For this review, take the finished solid that the model builds, in its own axes (mm). Face numbers are marked on the shaded views. A direction names the side the tool comes from. Round coordinates to 2 decimals unless told otherwise and drop trailing zeros. Order: outer loops, then holes, each group sorted by start corner. A loop starts at its lowest first (then second) coordinate and runs counter-clockwise, first axis right, second up.
from build123d import *

# Parameters (mm, degrees)
SKETCH1_W           = 60.861702088
SKETCH1_H           = 96.997143498
BOSS_EXTRUDE1_DEPTH = 50
SKETCH2_W           = 54.597089422
SKETCH2_H           = 86.84373193
CUT_EXTRUDE1_DEPTH  = 50
SKETCH3_R           = 4.118180668
SKETCH3_R_2         = 4.272844434
SKETCH3_R_3         = 3.932739474
CUT_EXTRUDE2_DEPTH  = 6
SKETCH4_R           = 3.08771087
BOSS_EXTRUDE2_DEPTH = 2
SKETCH5_R           = 2.038212953
CUT_EXTRUDE3_DEPTH  = 2
SKETCH6_R           = 3.908744467
SKETCH6_R_2         = 2.535125685
BOSS_EXTRUDE3_DEPTH = 2
SKETCH7_R           = 2.219432532
CUT_EXTRUDE4_DEPTH  = 2
SKETCH8_W           = 47.395397398
SKETCH8_H           = 4.29160036
SKETCH8_W_2         = 46.234961005
SKETCH8_H_2         = 3.842331126
SKETCH8_W_3         = 46.458453643
SKETCH8_H_3         = 4.013838195
SKETCH8_W_4         = 44.816524007
SKETCH8_H_4         = 3.759016324
SKETCH8_W_5         = 44.332896866
SKETCH8_H_5         = 3.544111845
SKETCH8_W_6         = 43.835439371
SKETCH8_H_6         = 4.852900567
SKETCH8_W_7         = 44.232019009
SKETCH8_H_7         = 3.586032373
SKETCH8_W_8         = 44.502323157
SKETCH8_H_8         = 5.537324529
BOSS_EXTRUDE4_DEPTH = 2
SKETCH9_W           = 44.730161392
SKETCH9_H           = 4.206770637
SKETCH9_W_2         = 43.731962655
SKETCH9_H_2         = 4.51977805
BOSS_EXTRUDE5_DEPTH = 2


with BuildPart() as part:
    # Sketch1 → Boss-Extrude1 (new body)
    with BuildSketch(Plane.XY):
        Rectangle(SKETCH1_W, SKETCH1_H)
    extrude(amount=BOSS_EXTRUDE1_DEPTH)

    # Sketch2 → Cut-Extrude1 (cut)
    with BuildSketch(Plane.XY.offset(50)):
        with Locations((-0.054476232, 0.453696841)):
            Rectangle(SKETCH2_W, SKETCH2_H)
    extrude(amount=-CUT_EXTRUDE1_DEPTH, mode=Mode.SUBTRACT)

    # Sketch3 → Cut-Extrude2 (cut)
    with BuildSketch(Plane(origin=(0, 48.498571749, 0), x_dir=(1, 0, 0), z_dir=(0, 1, 0))):
        with Locations(Location((-17.379612091, -22.981855157, 0), (0, 0, 270))):
            Circle(SKETCH3_R)
        with Locations(Location((0.816264726, -22.981855157, 0), (0, 0, 270))):
            Circle(SKETCH3_R_2)
        with Locations(Location((18.098885302, -22.981855157, 0), (0, 0, 270))):
            Circle(SKETCH3_R_3)
    extrude(amount=-CUT_EXTRUDE2_DEPTH, mode=Mode.SUBTRACT)

    # Sketch4 → Boss-Extrude2 (add)
    with BuildSketch(Plane(origin=(30.430851044, 0, 0), x_dir=(0, 0, -1), z_dir=(1, 0, 0))):
        with Locations(Location((-14.163441472, 33.849346779, 0), (0, 0, 180))):
            Circle(SKETCH4_R)
    extrude(amount=BOSS_EXTRUDE2_DEPTH)

    # Sketch5 → Cut-Extrude3 (cut)
    with BuildSketch(Plane(origin=(32.430851044, 0, 0), x_dir=(0, 0, -1), z_dir=(1, 0, 0))):
        with Locations((-13.96185256, 33.734367255)):
            Circle(SKETCH5_R)
    extrude(amount=-CUT_EXTRUDE3_DEPTH, mode=Mode.SUBTRACT)

    # Sketch6 → Boss-Extrude3 (add)
    with BuildSketch(Plane.ZY.offset(30.430851044)):
        with Locations(Location((13.179644946, 35.995992558, 0), (0, 0, 180))):
            Circle(SKETCH6_R)
        with Locations((13.179644946, 35.995992558)):
            Circle(SKETCH6_R_2, mode=Mode.SUBTRACT)
    extrude(amount=BOSS_EXTRUDE3_DEPTH)

    # Sketch7 → Cut-Extrude4 (cut)
    with BuildSketch(Plane.ZY.offset(30.430851044)):
        with Locations((13.179644946, 35.995992558)):
            Circle(SKETCH7_R)
    extrude(amount=-CUT_EXTRUDE4_DEPTH, mode=Mode.SUBTRACT)

    # Sketch8 → Boss-Extrude4 (add)
    with BuildSketch(Plane.ZY.offset(-27.244068479)):
        with Locations((24.521897503, 28.206728859)):
            Rectangle(SKETCH8_W, SKETCH8_H)
        with Locations((25.229689805, 18.94599963)):
            Rectangle(SKETCH8_W_2, SKETCH8_H_2)
        with Locations((25.229689805, 10.788271288)):
            Rectangle(SKETCH8_W_3, SKETCH8_H_3)
        with Locations((23.657759327, 2.882970932)):
            Rectangle(SKETCH8_W_4, SKETCH8_H_4)
        with Locations((23.899572897, -5.013591611)):
            Rectangle(SKETCH8_W_5, SKETCH8_H_5)
        with Locations((24.148301645, -13.789703554)):
            Rectangle(SKETCH8_W_6, SKETCH8_H_6)
        with Locations((23.950011826, -21.862272303)):
            Rectangle(SKETCH8_W_7, SKETCH8_H_7)
        with Locations((24.1320976, -31.257152078)):
            Rectangle(SKETCH8_W_8, SKETCH8_H_8)
    extrude(amount=BOSS_EXTRUDE4_DEPTH)

    # Sketch9 → Boss-Extrude5 (add)
    with BuildSketch(Plane.ZY.offset(-27.244068479)):
        with Locations((24.880043499, 35.759572617)):
            Rectangle(SKETCH9_W, SKETCH9_H)
        with Locations((23.711117662, -38.822738944)):
            Rectangle(SKETCH9_W_2, SKETCH9_H_2)
    extrude(amount=BOSS_EXTRUDE5_DEPTH)


solid = part.part
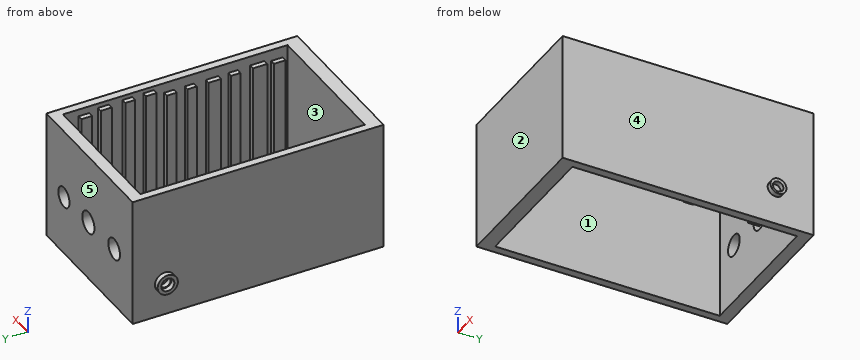
(1) Clearance check with flat-ended pins moving along their axes: P1, Ø2, axis at x = 26, y = 28, coming from the +Z side; P2, Ø4.5, axis at y = -30.5, z = 23.5, coming from the -X side; P3, Ø1, axis at x = 26.5, y = -39.5, coming from the -Z side. State where each tip first meets the part, or that it passes through.
(2) Tool access review of the marked faces 1 and 2: name each direction out of +Z, -Z, +X, -X, +Y, -Y from which nothing blocks a thin tool from reaching the whole face with its end or side.
(3) Wall thickness on L1, parallel to Y at x = 23, z = 41; L2, parallel to X at y = 10, z = 44.5; L3, parallel to X at y = -7, z = 37: over which ranges is each line inside the solid? List them lowest first.
(4) Add section B-B on x = -8. Give the boundary of the cut face in (y, z).
(5) Add section A-A on y = 24.5. Give the boundary of the cut face in (x, z).
(6) Add section D-D on x = -16. Give the boundary of the cut face in (y, z), plus the area to 3 significant figures.
(7) Add section C-C on y = -14. Give the boundary of the cut face in (x, z).
(8) Draft analysis for pull direction Y (two halves, no side actions). For the marked faces 3, 4 and 5, state which applies: pulls with the +Y half, pulls with the -Y half, needs draft (parallel to the pull), parting line crosses it, or undercut.
Here are the results:
1. P1: stops at z = 48.22
1. P2: stops at x = -30.43
1. P3: stops at z = 1.85
2. face 1: +Z, -Z
2. face 2: +Z, -Z, +X, -X, -Y
3. L1: y = -48.5 to -42.97, 43.88 to 48.5
3. L2: x = -30.43 to -27.35, 25.24 to 30.43
3. L3: x = -30.43 to -27.35, 27.24 to 30.43
4. outline: (-48.5, 0) - (-42.97, 0) - (-42.97, 50) - (-48.5, 50) - close; (43.88, 0) - (48.5, 0) - (48.5, 50) - (43.88, 50) - close
5. outline: (-30.43, 0) - (-27.35, 0) - (-27.35, 50) - (-30.43, 50) - close; (27.24, 0) - (30.43, 0) - (30.43, 50) - (27.24, 50) - close
6. outline: (-48.5, 0) - (-42.97, 0) - (-42.97, 50) - (-48.5, 50) - close; (43.88, 0) - (48.5, 0) - (48.5, 19.1) - (43.88, 19.1) - close; (43.88, 26.86) - (48.5, 26.86) - (48.5, 50) - (43.88, 50) - close
6. area: 472 mm2
7. outline: (-30.43, 0) - (-27.35, 0) - (-27.35, 50) - (-30.43, 50) - close; (25.24, 2.23) - (27.24, 2.23) - (27.24, 0) - (30.43, 0) - (30.43, 50) - (27.24, 50) - (27.24, 46.07) - (25.24, 46.07) - close
8. face 3: undercut
8. face 4: needs draft
8. face 5: pulls with the +Y half
